Design review of the part built by this model. Coordinates are the model's own, in mm. A direction names the side the tool comes from. Round coordinates to 2 decimals unless told otherwise and drop trailing zeros. Loops run counter-clockwise (first coordinate to the right, second up) from the corner with the lowest first, then second, coordinate; pieces in that order, holes last. Notation, with made-up numbers: (2.5, 81) - (36.5, 81) arc R19 ccw to (36.5, 92) - close; hole circle Ø8 at (77, 5). An arc over 180 degrees is marked (long way). Return JSON: item names as keys, results as strings. Group by question number.
(1) The part is to be moulded in two halves that separate along X. For faces 1 (the flat face through (140.769, 52, 0)), 2 (the flat face through (-129.231, 46, 0)), 3 (the flat face through (13, -150.769, 0)), say which applies: pulls with the +X half, pulls with the -X half, needs draft (parallel to the pull), parting line crosses it, or undercut.
(2) For faces 4 (the flat face through (-119.231, 47, 0)), 5 (the flat face through (-125, 50, -5)), list the 3-axis set-ups (+Z, -Z, +X, -X, +Y, -Y) from which the entire face can be reached by the end or side of a thin tool; tool diameter is ignored.
(3) We need section B-B, the plane x = -24. Write out the cut boundary in (y, z), and give its area (3 significant figures).
(4) Wall thickness on L1, parallel to X at y = 84.5, z = 2; L2, parallel to Y at x = 55, z = 2.5: over which ranges is each line inside the solid? List them lowest first. Write a range as [from, to].
(5) We need section C-C, the plane z = 0. Write out the cut boundary in (x, y), and give its area (3 significant figures).
(6) We need section A-A, the plane y = -17. Write out the cut boundary in (x, z).
Autodesk Inventor part; units mm, degrees
ref_plane "YZ Plane" through (0, 0, 0) normal (1, 0, 0) x (0, 1, 0)
ref_plane "XZ Plane" through (0, 0, 0) normal (0, 1, 0) x (-1, 0, 0)
ref_plane "XY Plane" through (0, 0, 0) normal (0, 0, 1) x (1, 0, 0)
sketch "Sketch1" plane through (0, 0, 0) normal (0, 0, 1) x (1, 0, 0)
  line L0 (-129.2308, 249.2308) -> (150.7692, 249.2308)
  line L1 (150.7692, 249.2308) -> (150.7692, -150.7692)
  line L2 (150.7692, -150.7692) -> (-129.2308, -150.7692)
  line L3 (-129.2308, -150.7692) -> (-129.2308, 249.2308)
  line L4 (-119.2308, 239.2308) -> (140.7692, 239.2308)
  line L5 (140.7692, 239.2308) -> (140.7692, -140.7692)
  line L6 (140.7692, -140.7692) -> (-119.2308, -140.7692)
  line L7 (-119.2308, -140.7692) -> (-119.2308, 239.2308)
  point P0 (0, 0)
  dimension "d0" = 280
  dimension "d1" = 400
  dimension "d2" = 10
  dimension "d3" = 10
  dimension "d4" = 10
  dimension "d5" = 10
  dimension "d6" = 150.7692
  dimension "d7" = 249.2308
extrude "Extrusion1" add sketch "Sketch1" along normal mid plane 10
properties part number "Steel support 5" material "Steel"
Solutions:
{
 "1": {"face 1": "undercut", "face 2": "pulls with the -X half", "face 3": "needs draft"},
 "2": {"face 4": "+Z, -Z", "face 5": "-Z, +X, -X, +Y, -Y"},
 "3": {"outline": "(-150.77, -5) - (-140.77, -5) - (-140.77, 5) - (-150.77, 5) - close; (239.23, -5) - (249.23, -5) - (249.23, 5) - (239.23, 5) - close", "area": "200 mm^2"},
 "4": {"L1": "[-129.23, -119.23], [140.77, 150.77]", "L2": "[-150.77, -140.77], [239.23, 249.23]"},
 "5": {"outline": "(-129.23, -150.77) - (150.77, -150.77) - (150.77, 249.23) - (-129.23, 249.23) - close; hole (-119.23, -140.77) - (140.77, -140.77) - (140.77, 239.23) - (-119.23, 239.23) - close", "area": "13,200 mm^2"},
 "6": {"outline": "(-129.23, -5) - (-119.23, -5) - (-119.23, 5) - (-129.23, 5) - close; (140.77, -5) - (150.77, -5) - (150.77, 5) - (140.77, 5) - close"}
}
